from build123d import *

# Parameters (mm, degrees)
F0_R     = 5
F1_DEPTH = 15
F0_W     = 30
F0_H     = 30
F2_DEPTH = 5
F4_D     = 2.5
F4_DEPTH = 10
F4_TIP   = 0.7510757738


with BuildPart() as f1:
    # F0 (on Top) → F1 (new body)
    with BuildSketch(Plane.XY):
        Circle(F0_R)
    extrude(amount=-F1_DEPTH)

    # F0 (on Top) → F2 (join)
    with BuildSketch(Plane.XY):
        Rectangle(F0_W, F0_H)
        Circle(F0_R, mode=Mode.SUBTRACT)
    extrude(amount=-F2_DEPTH)

    # F4
    with Locations(Plane(origin=(0, 0, -15), x_dir=(1, 0, 0), z_dir=(0, 0, -1))):
        with Locations((0, 0)):
            Hole(F4_D / 2, depth=F4_DEPTH)
            with Locations((0, 0, -(F4_DEPTH + F4_TIP / 2))):  # 118° drill point
                Cone(0, F4_D / 2, F4_TIP, mode=Mode.SUBTRACT)


solid = f1.part
CAD build for the part. Positions are in the model's coordinates, mm. A direction names the side the tool comes from. Round coordinates to 2 decimals unless told otherwise and drop trailing zeros. Write each loop counter-clockwise with the first axis right and the second up, starting at its lowest first coordinate (ties: lowest second). Pieces come first, ordered by that corner, then holes.
(1) Drop flat-ended pins along their axis: P1, Ø5, axis at x = -6, z = -12.5, coming from the -Y side; P2, Ø2, axis at x = 8, y = 7, coming from the -Z side; P3, Ø2, axis at y = -8.5, z = -7.5, coming from the -X side; P4, Ø2, axis at x = 0, y = 0, coming from the -Z side. Give the stop position or say it passes through.
(2) 3-axis set-ups, long thin cutter, end or side, ignore diameter. For faces 1 (the face through (1, -1, -15)), 2 (the face through (-1.08, -4.88, -9.93)): which of +Z, -Z, +X, -X, +Y, -Y reach the whole face in a straight line?
(3) Probe line 1 along Y through (x, z) = (0, -9.5); line 2 along Z through (x, y) = (5.25, -4.5); line 3 along X through (y, z) = (-0.75, -5.25). List the from-to ranges inside material, lowest first.
(4) Slice it at D-D, the plane y = -4.25. Write the cut outline in (x, z).
(5) Slice it at A-A, the plane z = -7.5. Write the cut outline in (x, y).
(6) Mould opens along X. For faces 3 (the face through (0.27, 1.22, -9.93)), 4 (the face through (-15, 0, -2)), 5 (the face through (0, 15, -2)), 6 (the face through (-0.05, 0.21, -4.38)) say: pulls with the +X half, pulls with the -X half, needs draft (parallel to the pull), parting line crosses it, or undercut.
(7) Slice it at B-B, the plane y = 12.5. Write the cut outline in (x, z), and give its area (3 significant figures).
From the geometry:
1. P1: stops at y = -3.57
1. P2: stops at z = -5
1. P3: passes through
1. P4: stops at z = -4.85
2. face 1: -Z, +X, -X, +Y, -Y
2. face 2: -Z
3. line 1: y = -5 to -1.25, 1.25 to 5
3. line 2: z = -5 to 0
3. line 3: x = -4.94 to -1, 1 to 4.94
4. outline: (-15, -5) - (-2.63, -5) - (-2.63, -15) - (2.63, -15) - (2.63, -5) - (15, -5) - (15, 0) - (-15, 0) - close
5. outline: circle Ø10 at (0, 0); hole circle Ø2.5 at (0, 0)
6. face 3: undercut
6. face 4: pulls with the -X half
6. face 5: needs draft
6. face 6: undercut
7. outline: (-15, -5) - (15, -5) - (15, 0) - (-15, 0) - close
7. area: 150 mm2
